from build123d import *

# Parameters (mm, degrees)
SKETCH1_R           = 57.5
BOSS_EXTRUDE1_DEPTH = 33.6
SKETCH2_R           = 50
CUT_EXTRUDE1_DEPTH  = 28.6
SKETCH3_R           = 2
SKETCH3_R_2         = 15
CUT_EXTRUDE2_DEPTH  = 31.8
SKETCH4_R           = 1.75
SKETCH4_R_2         = 1.5
CUT_EXTRUDE3_DEPTH  = 50
SKETCH9_W           = 40
SKETCH9_H           = 28.6
CUT_EXTRUDE4_DEPTH  = 72
CIRPATTERN1_COUNT   = 4
FILLET2_R           = 5
CHAMFER1_SIZE       = 5


with BuildPart() as part:
    # Sketch1 → Boss-Extrude1 (new body)
    with BuildSketch(Plane(origin=(0, 0, 0), x_dir=(1, 0, 0), z_dir=(0, 1, 0))):
        with Locations(Location((0, 0, 0), (0, 0, 270))):
            Circle(SKETCH1_R)
    extrude(amount=BOSS_EXTRUDE1_DEPTH)

    # Sketch2 → Cut-Extrude1 (cut)
    with BuildSketch(Plane(origin=(0, 33.6, 0), x_dir=(1, 0, 0), z_dir=(0, 1, 0))):
        with Locations(Location((0, 0, 0), (0, 0, 270))):
            Circle(SKETCH2_R)
    extrude(amount=-CUT_EXTRUDE1_DEPTH, mode=Mode.SUBTRACT)

    # Sketch3 → Cut-Extrude2 (cut)
    with BuildSketch(Plane.XZ):
        with BuildLine():
            Line((-10, 25.617376915), (-10, 43.874821937))
            ThreePointArc((-10, 43.874821937), (-31.819805153, 31.819805153), (-43.874821937, 10))
            Line((-43.874821937, 10), (-25.617376915, 10))
            ThreePointArc((-25.617376915, 10), (-19.445436483, 19.445436483), (-10, 25.617376915))
        make_face()
        with BuildLine():
            Line((25.617376915, 10), (43.874821937, 10))
            ThreePointArc((43.874821937, 10), (31.819805153, 31.819805153), (10, 43.874821937))
            Line((10, 43.874821937), (10, 25.617376915))
            ThreePointArc((10, 25.617376915), (19.445436483, 19.445436483), (25.617376915, 10))
        make_face()
        with BuildLine():
            ThreePointArc((10, -43.874821937), (31.819805153, -31.819805153), (43.874821937, -10))
            Line((43.874821937, -10), (25.617376915, -10))
            ThreePointArc((25.617376915, -10), (19.445436483, -19.445436483), (10, -25.617376915))
            Line((10, -25.617376915), (10, -43.874821937))
        make_face()
        with BuildLine():
            ThreePointArc((-43.874821937, -10), (-31.819805153, -31.819805153), (-10, -43.874821937))
            Line((-10, -43.874821937), (-10, -25.617376915))
            ThreePointArc((-10, -25.617376915), (-19.445436483, -19.445436483), (-25.617376915, -10))
            Line((-25.617376915, -10), (-43.874821937, -10))
        make_face()
        with Locations(Location((-20, 0, 0), (0, 0, 270))):
            Circle(SKETCH3_R)
        with Locations(Location((0, 0, 0), (0, 0, 270))):
            Circle(SKETCH3_R_2)
        with Locations(Location((0, 20, 0), (0, 0, 270))):
            Circle(SKETCH3_R)
        with Locations(Location((20, 0, 0), (0, 0, 270))):
            Circle(SKETCH3_R)
        with Locations(Location((0, -20, 0), (0, 0, 270))):
            Circle(SKETCH3_R)
    extrude(amount=-CUT_EXTRUDE2_DEPTH, mode=Mode.SUBTRACT)

    # Sketch4 → Cut-Extrude3 (cut)
    with BuildSketch(Plane.XZ):
        with Locations(Location((0, 54, 0), (0, 0, 270))):
            Circle(SKETCH4_R)
        with Locations(Location((27, 46.765371804, 0), (0, 0, 270))):
            Circle(SKETCH4_R)
        with Locations(Location((46.765371804, 27, 0), (0, 0, 270))):
            Circle(SKETCH4_R)
        with Locations(Location((54, 0, 0), (0, 0, 270))):
            Circle(SKETCH4_R)
        with Locations(Location((46.765371804, -27, 0), (0, 0, 270))):
            Circle(SKETCH4_R)
        with Locations(Location((27, -46.765371804, 0), (0, 0, 270))):
            Circle(SKETCH4_R)
        with Locations(Location((0, -54, 0), (0, 0, 270))):
            Circle(SKETCH4_R)
        with Locations(Location((-27, -46.765371804, 0), (0, 0, 270))):
            Circle(SKETCH4_R)
        with Locations(Location((-46.765371804, -27, 0), (0, 0, 270))):
            Circle(SKETCH4_R)
        with Locations(Location((-54, 0, 0), (0, 0, 270))):
            Circle(SKETCH4_R)
        with Locations(Location((-46.765371804, 27, 0), (0, 0, 270))):
            Circle(SKETCH4_R)
        with Locations(Location((-27, 46.765371804, 0), (0, 0, 270))):
            Circle(SKETCH4_R)
        with Locations(Location((0, 30.405591591, 0), (0, 0, 270))):
            Circle(SKETCH4_R_2)
        with Locations(Location((30.405591591, 0, 0), (0, 0, 270))):
            Circle(SKETCH4_R_2)
        with Locations(Location((0, -30.405591591, 0), (0, 0, 270))):
            Circle(SKETCH4_R_2)
        with Locations(Location((-30.405591591, 0, 0), (0, 0, 270))):
            Circle(SKETCH4_R_2)
    extrude(amount=-CUT_EXTRUDE3_DEPTH, mode=Mode.SUBTRACT)

    # Sketch9 → Cut-Extrude4 (cut)
    with BuildSketch(Plane.XY):
        with Locations((0, 19.3)):
            Rectangle(SKETCH9_W, SKETCH9_H)
    cut_extrude4 = extrude(amount=-CUT_EXTRUDE4_DEPTH, mode=Mode.SUBTRACT)

    # CirPattern1: Cut-Extrude4 ×4 about axis
    cirpattern1_axis = Axis((0, 0, 0), (0, 1, 0))
    for i in range(1, CIRPATTERN1_COUNT):
        add(cut_extrude4.rotate(cirpattern1_axis, i * 360 / CIRPATTERN1_COUNT), mode=Mode.SUBTRACT)

    # Fillet2
    fillet2_edges = [part.edges().sort_by_distance(p)[0] for p in [
        (43.874821937, 2.5, 10),
        (25.617376915, 2.5, 10),
        (10, 2.5, 25.617376915),
        (10, 2.5, 43.874821937),
        (10, 2.5, -43.874821937),
        (10, 2.5, -25.617376915),
        (25.617376915, 2.5, -10),
        (43.874821937, 2.5, -10),
        (-43.874821937, 2.5, -10),
        (-25.617376915, 2.5, -10),
        (-10, 2.5, -25.617376915),
        (-10, 2.5, -43.874821937),
        (-10, 2.5, 43.874821937),
        (-10, 2.5, 25.617376915),
        (-25.617376915, 2.5, 10),
        (-43.874821937, 2.5, 10),
    ]]
    fillet(fillet2_edges, radius=FILLET2_R)

    # Chamfer1
    chamfer1_edges = [part.edges().sort_by_distance(p)[0] for p in [
        (-35.355339059, 5, -35.355339059),
        (-20, 5, -49.867701791),
        (20, 5, -49.867701791),
        (-35.355339059, 5, 35.355339059),
        (35.355339059, 5, 35.355339059),
        (35.355339059, 5, -35.355339059),
        (-49.867701791, 5, 20),
        (20, 5, 49.867701791),
        (49.867701791, 5, -20),
        (49.867701791, 5, 20),
        (-20, 5, 49.867701791),
        (-49.867701791, 5, -20),
    ]]
    chamfer(chamfer1_edges, length=CHAMFER1_SIZE - 0.0001)  # a hair under: the kernel refuses the full size


solid = part.part
Design review of the part built by this model. Coordinates are the model's own, in mm. A direction names the side the tool comes from. Give positions to 0.01 mm unless a question says otherwise; leave off trailing zeros. Write each loop counter-clockwise with the first axis right and the second up, starting at its lowest first coordinate (ties: lowest second). Pieces come first, ordered by that corner, then holes. Notation, with made-up numbers: M -16.5,-2 L -11.5,-2 A34 cw -11.5,30 Z; hole C -3.5,18.5 d1. An arc over 180 degrees is marked long. Return JSON: item names as keys, results as strings. Group by question number.
Item 1: Tool access review of faces 1 (the flat face through (-38, 33.6, 37)), 2 (the cylindrical face through (-12.262, 2.535, 41.265)): name each direction out of +Z, -Z, +X, -X, +Y, -Y from which nothing blocks a thin tool from reaching the whole face with its end or side.
Item 2: The part is to be moulded in two halves that separate along Z. For faces 3 (the flat face through (18, 8, -49)), 4 (the cylindrical face through (-22.023, 16.565, 53.115)), 5 (the cylindrical face through (-55.71, 2.46, 0.38)), say which applies: pulls with the +Z half, pulls with the -Z half, needs draft (parallel to the pull), parting line crosses it, or undercut.
Item 3: Wall thickness on line 1 along X through (y, z) = (4, -17); line 2 along X through (y, z) = (17.5, 27.5); line 3 along X through (y, z) = (26, -26.5): over which ranges is each line inside the solid? List them lowest first.
Item 4: Take a section at A-A (y = 17). Count the separate pieces of the cut face and the enclosed holes in it, plus the area to 3 significant figures.
Item 5: Clearance check with flat-ended pins moving along their axes: pin 1 Ø5.5 at (y, z) = (3.5, -34.5) entering from -X; pin 2 Ø2.5 at (y, z) = (1.5, 32) entering from +X; pin 3 Ø8 at (y, z) = (9.5, -45.5) entering from -X. State where each tip first meets the part, or that it passes through.
Item 6: Take a section at C-C (z = 8.5). Give the boundary of the cut face in (x, y), plus the area to 3 significant figures.
Return value:
{
 "1": {"face 1": "+Z, -Z, +X, -X, +Y", "face 2": "+Y, -Y"},
 "2": {"face 3": "needs draft", "face 4": "parting line crosses it", "face 5": "undercut"},
 "3": {"line 1": "x = -54.93 to -41.67, -21.62 to 21.62, 41.67 to 54.93", "line 2": "x = -50.5 to -48.44, -45.09 to -41.76, 41.76 to 45.09, 48.44 to 50.5", "line 3": "x = -51.03 to -48.44, -45.09 to -42.4, 42.4 to 45.09, 48.44 to 51.03"},
 "4": {"separate pieces": "4", "enclosed holes": "8", "area": "1,230 mm2"},
 "5": {"pin 1": "stops at x = -47.94", "pin 2": "stops at x = 48.59", "pin 3": "stops at x = -39.8"},
 "6": {"outline": "M -56.87,0 L -12.36,0 L -12.36,5 L -56.87,5 Z; M 12.36,0 L 56.87,0 L 56.87,5 L 12.36,5 Z", "area": "445 mm2"}
}
